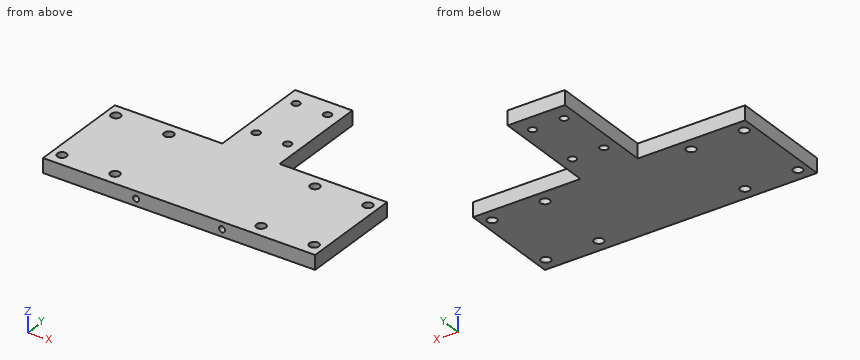
```python
from build123d import *

# Parameters (mm, degrees)
SKETCH_W               = 190
SKETCH_H               = 72
PAD_DEPTH              = 10
SKETCH001_W            = 40
SKETCH001_H            = 10
PAD001_DEPTH           = 73
SKETCH002_R            = 3.3
HOLE_DEPTH             = 10.001
LINEARPATTERN_COUNT    = 2
LINEARPATTERN_PITCH    = 37
LINEARPATTERN001_COUNT = 2
LINEARPATTERN001_PITCH = 139
LINEARPATTERN002_COUNT = 2
LINEARPATTERN002_PITCH = 176
SKETCH003_R            = 3.3
HOLE001_DEPTH          = 10.001
LINEARPATTERN003_COUNT = 2
LINEARPATTERN003_PITCH = 37
LINEARPATTERN004_COUNT = 2
LINEARPATTERN004_PITCH = 139
LINEARPATTERN005_COUNT = 2
LINEARPATTERN005_PITCH = 176
SKETCH004_R            = 2.75
HOLE002_DEPTH          = 10.001
LINEARPATTERN006_COUNT = 2
LINEARPATTERN006_PITCH = 22
LINEARPATTERN007_COUNT = 2
LINEARPATTERN007_PITCH = 40
SKETCH005_R            = 2.75
HOLE003_DEPTH          = 10.001
SKETCH006_R            = 2.1
HOLE004_DEPTH          = 25
LINEARPATTERN008_COUNT = 2
LINEARPATTERN008_PITCH = 60


with BuildPart() as part:
    # Sketch → Pad (new body)
    with BuildSketch(Plane.XY):
        with Locations((95, 36)):
            Rectangle(SKETCH_W, SKETCH_H)
    extrude(amount=PAD_DEPTH)

    # Sketch001 (on Face3 of Pad) → Pad001 (join)
    with BuildSketch(Plane(origin=(0, 72, 0), x_dir=(-1, 0, 0), z_dir=(0, 1, 0))):
        with Locations((-95, 5)):
            Rectangle(SKETCH001_W, SKETCH001_H)
    extrude(amount=PAD001_DEPTH)

    # Sketch002 (on Face5 of Pad001) → Hole (cut, through all)
    with BuildSketch(Plane.XY.offset(10)):
        with Locations((7, 9)):
            Circle(SKETCH002_R)
    hole = extrude(amount=-HOLE_DEPTH, mode=Mode.SUBTRACT)

    # LinearPattern: Hole ×2
    with Locations(*[(i * LINEARPATTERN_PITCH, 0, 0) for i in range(1, LINEARPATTERN_COUNT)]):
        add(hole, mode=Mode.SUBTRACT)

    # LinearPattern001: Hole ×2
    with Locations(*[(i * LINEARPATTERN001_PITCH, 0, 0) for i in range(1, LINEARPATTERN001_COUNT)]):
        add(hole, mode=Mode.SUBTRACT)

    # LinearPattern002: Hole ×2
    with Locations(*[(i * LINEARPATTERN002_PITCH, 0, 0) for i in range(1, LINEARPATTERN002_COUNT)]):
        add(hole, mode=Mode.SUBTRACT)

    # Sketch003 (on Face5 of LinearPattern002) → Hole001 (cut, through all)
    with BuildSketch(Plane.XY.offset(10)):
        with Locations((7, 63)):
            Circle(SKETCH003_R)
    hole001 = extrude(amount=-HOLE001_DEPTH, mode=Mode.SUBTRACT)

    # LinearPattern003: Hole001 ×2
    with Locations(*[(i * LINEARPATTERN003_PITCH, 0, 0) for i in range(1, LINEARPATTERN003_COUNT)]):
        add(hole001, mode=Mode.SUBTRACT)

    # LinearPattern004: Hole001 ×2
    with Locations(*[(i * LINEARPATTERN004_PITCH, 0, 0) for i in range(1, LINEARPATTERN004_COUNT)]):
        add(hole001, mode=Mode.SUBTRACT)

    # LinearPattern005: Hole001 ×2
    with Locations(*[(i * LINEARPATTERN005_PITCH, 0, 0) for i in range(1, LINEARPATTERN005_COUNT)]):
        add(hole001, mode=Mode.SUBTRACT)

    # Sketch004 (on Face17 of LinearPattern005) → Hole002 (cut, through all)
    with BuildSketch(Plane.XY.offset(10)):
        with Locations((84, 93)):
            Circle(SKETCH004_R)
    hole002 = extrude(amount=-HOLE002_DEPTH, mode=Mode.SUBTRACT)

    # LinearPattern006: Hole002 ×2
    with Locations(*[(i * LINEARPATTERN006_PITCH, 0, 0) for i in range(1, LINEARPATTERN006_COUNT)]):
        add(hole002, mode=Mode.SUBTRACT)

    # LinearPattern007: Hole002 ×2
    with Locations(*[(0, i * LINEARPATTERN007_PITCH, 0) for i in range(1, LINEARPATTERN007_COUNT)]):
        add(hole002, mode=Mode.SUBTRACT)

    # Sketch005 (on Face17 of LinearPattern007) → Hole003 (cut, through all)
    with BuildSketch(Plane.XY.offset(10)):
        with Locations((106, 133)):
            Circle(SKETCH005_R)
    extrude(amount=-HOLE003_DEPTH, mode=Mode.SUBTRACT)

    # Sketch006 (on Face1 of Hole003) → Hole004 (cut)
    with BuildSketch(Plane.XZ):
        with Locations((65, 5)):
            Circle(SKETCH006_R)
    hole004 = extrude(amount=-HOLE004_DEPTH, mode=Mode.SUBTRACT)

    # LinearPattern008: Hole004 ×2
    with Locations(*[(i * LINEARPATTERN008_PITCH, 0, 0) for i in range(1, LINEARPATTERN008_COUNT)]):
        add(hole004, mode=Mode.SUBTRACT)


solid = part.part
```
The listing builds one solid part. Answer for the finished solid, in the listing's coordinates (mm). Give positions to 0.01 mm unless a question says otherwise; leave off trailing zeros. Loops run counter-clockwise (first coordinate to the right, second up) from the corner with the lowest first, then second, coordinate; pieces in that order, holes last. Notation, with made-up numbers: (85.5, -34) - (140.5, -34) arc R22 cw to (140.5, -10) - close; hole circle Ø4 at (-17, 52.5). An arc over 180 degrees is marked (long way). Answer as CSV lines item,"result". Start each with the question number.
Item 1: Each of these flat-tipped pins is pushed along its axis until it touches: pin 1 (5.5 mm diameter, centred on x = 7, y = 63, fed in from -Z); pin 2 (1.3 mm diameter, centred on x = 124.5, z = 5.5, fed in from -Y); pin 3 (5 mm diameter, centred on y = 110, z = 4, fed in from -X); pin 4 (5 mm diameter, centred on y = 97.5, z = 8.5, fed in from +X). Where does it stop, or does it pass through?
Item 2: A cutting plane is placed at A-A on x = 106. Determine the outline of the cut face in (y, z), then the cut area to 3 significant figures.
Item 3: A cutting plane is placed at C-C on y = 133. Determine the outline of the cut face in (x, z), then the cut area to 3 significant figures.
Item 4: A cutting plane is placed at D-D on x = 65. Determine the outline of the cut face in (y, z).
Item 5: Find the intervals of material crossed by line 1 (Y direction, x = 146, z = 3.5); line 2 (X direction, y = 65, z = 6.5); line 3 (X direction, y = 64.5, z = 6), in increasing order. Write a range as from..to.
Item 6: A cutting plane is placed at B-B on z = 5. Count the separate pieces of the cut face and the enclosed holes in it, then the cut area to 3 significant figures.
Found:
1,pin 1,"passes through"
1,pin 2,"stops at y = 25"
1,pin 3,"stops at x = 75"
1,pin 4,"stops at x = 115"
2,outline,"(0, 0) - (90.25, 0) - (90.25, 10) - (0, 10) - close; (95.75, 0) - (130.25, 0) - (130.25, 10) - (95.75, 10) - close; (135.75, 0) - (145, 0) - (145, 10) - (135.75, 10) - close"
2,area,"1,340 mm^2"
3,outline,"(75, 0) - (81.25, 0) - (81.25, 10) - (75, 10) - close; (86.75, 0) - (103.25, 0) - (103.25, 10) - (86.75, 10) - close; (108.75, 0) - (115, 0) - (115, 10) - (108.75, 10) - close"
3,area,"290 mm^2"
4,outline,"(0, 0) - (72, 0) - (72, 10) - (0, 10) - (0, 7.1) - (25, 7.1) - (25, 2.9) - (0, 2.9) - close"
5,line 1,"y = 0..5.7, 12.3..59.7, 66.3..72"
5,line 2,"x = 0..4.38, 9.62..41.38, 46.62..143.38, 148.62..180.38, 185.62..190"
5,line 3,"x = 0..4.06, 9.94..41.06, 46.94..143.06, 148.94..180.06, 185.94..190"
6,separate pieces,"1"
6,enclosed holes,"12"
6,area,"16,000 mm^2"
